Geometry check sheet. Reference: the model listing, model coordinates, mm. A direction names the side the tool comes from. Coordinates: 2 decimals unless noted, no trailing zeros. Order: outer loops, then holes, each group sorted by start corner. A loop starts at its lowest first (then second) coordinate and runs counter-clockwise, first axis right, second up. Notation, with made-up numbers: M 57.25,-35 L 100.25,-35 A18 ccw 100.25,-21 Z; hole C 51.5,-21.75 d10. An arc over 180 degrees is marked long. Use CSV: the item, a comma, the result in double quotes. Start each with the question number.
```python
from build123d import *

# Parameters (mm, degrees)
F0_R     = 11.1125
F1_DEPTH = 6.35
F2_R     = 3.175
F3_DEPTH = 3.175
F4_R     = 3.175
F5_DEPTH = 3.175
F7_DEPTH = 25.4
F8_R     = 3.175
F9_DEPTH = 12.7


with BuildPart() as f1:
    # F0 (on Front) → F1 (new body, symmetric)
    with BuildSketch(Plane.XZ):
        Circle(F0_R)
    extrude(amount=F1_DEPTH, both=True)

    # F2 (on face) → F3 (join)
    with BuildSketch(Plane.XZ.offset(6.35)):
        Circle(F2_R)
    extrude(amount=F3_DEPTH)

    # F4 (on face) → F5 (join)
    with BuildSketch(Plane(origin=(0, 6.35, 0), x_dir=(-1, 0, 0), z_dir=(0, 1, 0))):
        Circle(F4_R)
    extrude(amount=F5_DEPTH)

    # F6 (on face) → F7 (cut)
    with BuildSketch(Plane(origin=(0, 9.525, 0), x_dir=(-1, 0, 0), z_dir=(0, 1, 0))):
        with BuildLine():
            ThreePointArc((-6.4359051175, 9.0590717829), (-11.1125, 0), (-6.4359051175, -9.0590717829))
            Line((-6.4359051175, -9.0590717829), (-6.4359051175, 9.0590717829))
        make_face()
    extrude(amount=-F7_DEPTH, mode=Mode.SUBTRACT)

    # F8 (on face) → F9 (cut)
    with BuildSketch(Plane.YZ.offset(6.4359051175)):
        Circle(F8_R)
    extrude(amount=-F9_DEPTH, mode=Mode.SUBTRACT)


solid = f1.part
```
1) Section check D-D on x = -10. Record the boundary of the cut face in (y, z).
2) Draft check along Z on faces 1 (the face through (-2.5, 6.35, -2.3)), 2 (the face through (-6.264, 0, 0)), 3 (the face through (-11.107, -0.089, 0.34)). Enter one of: +Z half, -Z half, draft (parallel to the pull), parting line (faces both ways), or undercut.
3) Set-up check for faces 4 (the face through (6.436, 3, 2)), 5 (the face through (0.69, 7.92, -3.1)), 6 (the face through (0.17, -0.69, -3.1)), 7 (the face through (-0.69, -7.92, -3.1)), 8 (the face through (0, 9.525, 0)): record each of +Z, -Z, +X, -X, +Y, -Y from which the full face is reachable in a straight line by a thin tool's end or side.
4) Gauge pin test, flat ends, axial feed: P1, Ø8.5, axis at y = 0, z = 0, coming from the +X side; P2, Ø1, axis at x = -4.5, z = 8.5, coming from the -Y side; P3, Ø3, axis at x = 1.5, z = 9, coming from the +Y side; P4, Ø3, axis at y = 2, z = -5, coming from the -X side. Record the tip position at first contact, or that the pin passes through.
5) Material ranges on line 1 along Z through (x, y) = (0.25, 0) (3 decimals); line 2 along Y through (x, z) = (-4, -3.75); line 3 along Z through (x, y) = (-2.5, 2.75), recorded low to high.
6) Section check C-C on y = 0. Record the boundary of the cut face in (x, z) (1 decimal).
Results are:
1,outline,"M -6.35,-4.85 L 6.35,-4.85 L 6.35,4.85 L -6.35,4.85 Z"
2,face 1,"draft"
2,face 2,"undercut"
2,face 3,"parting line"
3,face 4,"+Z, -Z, +X, +Y, -Y"
3,face 5,"+Y"
3,face 6,"+X"
3,face 7,"-Y"
3,face 8,"+Z, -Z, +X, -X, +Y"
4,P1,"stops at x = 6.44"
4,P2,"stops at y = -6.35"
4,P3,"stops at y = 6.35"
4,P4,"stops at x = -10.55"
5,line 1,"z = -11.11 to -3.175, 3.175 to 11.11"
5,line 2,"y = -6.35 to 6.35"
5,line 3,"z = -10.83 to -1.59, 1.59 to 10.83"
6,outline,"M -6.3,-3.2 L -6.3,3.2 L 6.4,3.2 L 6.4,9.1 A11.1 ccw long 6.4,-9.1 L 6.4,-3.2 Z"
